The model under review builds one solid part; all positions refer to its coordinate system, in mm. Face numbers are marked on the shaded views. A direction names the side the tool comes from. Give positions to 0.01 mm unless a question says otherwise; leave off trailing zeros. Write each loop counter-clockwise with the first axis right and the second up, starting at its lowest first coordinate (ties: lowest second). Pieces come first, ordered by that corner, then holes. Notation, with made-up numbers: (7.25, 45.5) -> (38.25, 45.5) arc R12 cw to (38.25, 67.5) -> close; hole circle Ø9 at (24.5, 73). An arc over 180 degrees is marked (long way). Use CSV: the item, a comma, the result in double quotes.
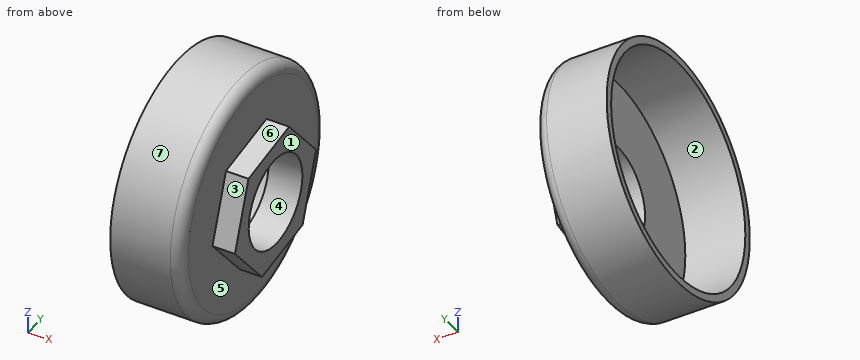
```python
from build123d import *

# Parameters (mm, degrees)
SKETCH1_R           = 32
BOSS_EXTRUDE1_DEPTH = 19
SKETCH5_R           = 30
CUT_EXTRUDE1_DEPTH  = 16
FILLET1_R           = 3
BOSS_EXTRUDE2_DEPTH = 6
SKETCH7_R           = 12
CUT_EXTRUDE2_DEPTH  = 26


with BuildPart() as part:
    # Sketch1 → Boss-Extrude1 (new body)
    with BuildSketch(Plane(origin=(0, 0, 0), x_dir=(0, 0, -1), z_dir=(1, 0, 0))):
        Circle(SKETCH1_R)
    extrude(amount=BOSS_EXTRUDE1_DEPTH)

    # Sketch5 → Cut-Extrude1 (cut)
    with BuildSketch(Plane.ZY):
        Circle(SKETCH5_R)
    extrude(amount=-CUT_EXTRUDE1_DEPTH, mode=Mode.SUBTRACT)

    # Fillet1
    fillet1_edges = [part.edges().sort_by_distance(p)[0] for p in [
        (19, 0, 32),
    ]]
    fillet(fillet1_edges, radius=FILLET1_R)

    # Sketch6 → Boss-Extrude2 (add)
    with BuildSketch(Plane(origin=(19, 0, 0), x_dir=(0, 0, -1), z_dir=(1, 0, 0))):
        Polygon((-17.454071761, 6.057120794), (-13.972656361, -12.087109147), (3.481415399, -18.144229941), (17.454071761, -6.057120794), (13.972656361, 12.087109147), (-3.481415399, 18.144229941), align=None)
    extrude(amount=BOSS_EXTRUDE2_DEPTH)

    # Sketch7 → Cut-Extrude2 (cut, through all)
    with BuildSketch(Plane(origin=(25, 0, 0), x_dir=(0, 0, -1), z_dir=(1, 0, 0))):
        Circle(SKETCH7_R)
    extrude(amount=-CUT_EXTRUDE2_DEPTH, mode=Mode.SUBTRACT)


solid = part.part
```
Q1. Consider section C-C (y = 0). Write out the cut boundary in (x, z), then the cut area to 3 significant figures.
Derived:
outline,"(0, -32) -> (16, -32) arc R3 ccw to (19, -29) -> (19, -16.29) -> (25, -16.29) -> (25, -12) -> (16, -12) -> (16, -30) -> (0, -30) -> close; (0, 30) -> (16, 30) -> (16, 12) -> (25, 12) -> (25, 16.29) -> (19, 16.29) -> (19, 29) arc R3 ccw to (16, 32) -> (0, 32) -> close"
area,"232 mm2"
Q2. Machinability: for the marked faces 1, 2 and 3, which of the approach directions +Z, -Z, +X, -X, +Y, -Y give a long, thin tool a straight path to every point of the face, cutting with its end or side? Answer none if there is none.
Derived:
face 1,"+Z, -Z, +X, +Y, -Y"
face 2,"-X"
face 3,"+Z, +X, -Y"
Q3. To check wall thickness, follow probe 1 along Y at (x, z) = (3.75, 0); probe 2 along X at (y, z) = (-16, -1.5); probe 3 along Y at (x, z) = (12, 20.5). State the ranges of each line that lie inside material, in increasing order.
Derived:
probe 1,"y = -32 to -30, 30 to 32"
probe 2,"x = 16 to 25"
probe 3,"y = -24.57 to -21.9, 21.9 to 24.57"
Q4. Consider section B-B (z = 0). Write out the cut boundary in (x, y).
Derived:
outline,"(0, -32) -> (16, -32) arc R3 ccw to (19, -29) -> (19, -16.94) -> (25, -16.94) -> (25, -12) -> (16, -12) -> (16, -30) -> (0, -30) -> close; (0, 30) -> (16, 30) -> (16, 12) -> (25, 12) -> (25, 16.94) -> (19, 16.94) -> (19, 29) arc R3 ccw to (16, 32) -> (0, 32) -> close"
Q5. The part is to be moulded in two halves that separate along Z. For the marked faces 4, 5, 6 and 7, say which applies: pulls with the +Z half, pulls with the -Z half, needs draft (parallel to the pull), parting line crosses it, or undercut.
Derived:
face 4,"undercut"
face 5,"needs draft"
face 6,"pulls with the +Z half"
face 7,"parting line crosses it"
Q6. Consider section D-D (x = 6.5). Write out the cut boundary in (y, z).
Derived:
outline,"circle Ø64 at (0, 0); hole circle Ø60 at (0, 0)"
Q7. Consider section A-A (x = 20). Write out the cut boundary in (y, z), then the cut area to 3 significant figures.
Derived:
outline,"(-18.14, -3.48) -> (-6.06, -17.45) -> (12.09, -13.97) -> (18.14, 3.48) -> (6.06, 17.45) -> (-12.09, 13.97) -> close; hole circle Ø24 at (0, 0)"
area,"434 mm2"
Q8. Insertion check: pin 1 (3 mm diameter, centred on y = -20.5, z = 12, fed in from -X); pin 2 (12 mm diameter, centred on x = 10.5, y = 17, fed in from -Z); pin 3 (10 mm diameter, centred on x = 2.5, y = 10, fed in from +Z). Each pin has a flat end and moves straight along its axis. Give the tip position at first contact, or say it passes through.
Derived:
pin 1,"stops at x = 16"
pin 2,"stops at z = -30.05"
pin 3,"stops at z = 31.61"
